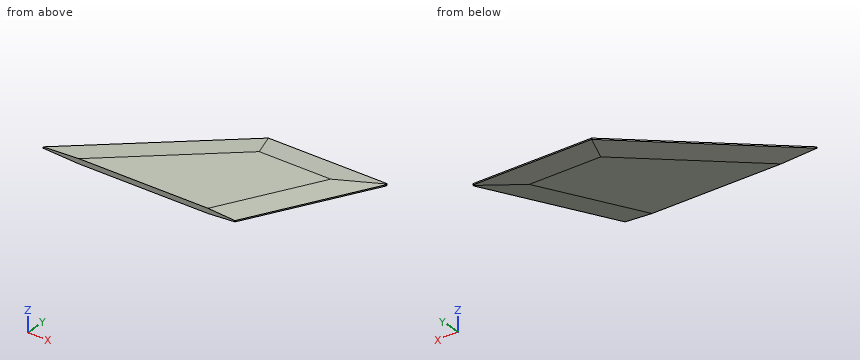
from build123d import *
from OCP.BRepFilletAPI import BRepFilletAPI_MakeChamfer

# Parameters (mm, degrees)
BOSS_EXTRUDE1_DEPTH = 1
CHAMFER1_SIZE       = 0.75
CHAMFER1_SIZE2      = 10
FILLET1_R           = 0.5


# Read off the part's stored shape, not the designer's step: Mirror1
with BuildPart() as part:
    # Sketch1 → Boss-Extrude1 (new, symmetric)
    with BuildSketch(Plane.XY):
        Polygon((0, 0), (80, 0), (105.530625741, 50), (55.530625741, 50), align=None)
    extrude(amount=BOSS_EXTRUDE1_DEPTH, both=True)

    # Chamfer1: one chamfer whose edges measure the first distance from different faces: ONE call of the kernel's chamfer builder (chamfer() names one face for all edges)
    chamfer1_edges_1 = [part.edges().sort_by_distance(p)[0] for p in [
        (92.765312871, 25, 1),
    ]]
    chamfer1_side_1 = [part.faces().sort_by_distance(p)[0] for p in [
        (92.765312871, 25, 0),
    ]]
    chamfer1_edges_2 = [part.edges().sort_by_distance(p)[0] for p in [
        (80.530625741, 50, 1),
    ]]
    chamfer1_side_2 = [part.faces().sort_by_distance(p)[0] for p in [
        (80.530625741, 50, 0),
    ]]
    chamfer1_edges_3 = [part.edges().sort_by_distance(p)[0] for p in [
        (27.765312871, 25, 1),
    ]]
    chamfer1_side_3 = [part.faces().sort_by_distance(p)[0] for p in [
        (27.765312871, 25, 0),
    ]]
    chamfer1 = BRepFilletAPI_MakeChamfer(part.part.solid().wrapped)
    for e in chamfer1_edges_1:
        chamfer1.Add(CHAMFER1_SIZE, CHAMFER1_SIZE2, e.wrapped, chamfer1_side_1[0].wrapped)  # the first distance lies on this face
    for e in chamfer1_edges_2:
        chamfer1.Add(CHAMFER1_SIZE, CHAMFER1_SIZE2, e.wrapped, chamfer1_side_2[0].wrapped)  # the first distance lies on this face
    for e in chamfer1_edges_3:
        chamfer1.Add(CHAMFER1_SIZE, CHAMFER1_SIZE2, e.wrapped, chamfer1_side_3[0].wrapped)  # the first distance lies on this face
    add(Compound.cast(chamfer1.Shape()), mode=Mode.REPLACE)

    # Mirror1
    split(bisect_by=Plane.XY, keep=Keep.TOP)

    # Mirror1 2: part across plane


with BuildPart() as part_1:
    add(part.part)
    add(part.part.mirror(Plane.XY))

    # Fillet1
    fillet1_edges = [part_1.edges().sort_by_distance(p)[0] for p in [
        (55.530625741, 50, 0),
        (105.530625741, 50, 0),
    ]]
    fillet(fillet1_edges, radius=FILLET1_R)


solid = part_1.part
The listing builds one solid part. Answer for the finished solid, in the listing's coordinates (mm). Coordinates: 2 decimals unless noted, no trailing zeros. Order: outer loops, then holes, each group sorted by start corner. A loop starts at its lowest first (then second) coordinate and runs counter-clockwise, first axis right, second up. Notation, with made-up numbers: (83, 2.5) -> (124, 2.5) arc R22 ccw to (124, 40.5) -> close; hole circle Ø11 at (65.5, 16.25). An arc over 180 degrees is marked (long way). Answer in a Markdown table with one row per item. Add a question column.
Item 1: Find section A-A (x = 72.5). Write down the section's boundary in (y, z).
Item 2: This flat-tipped pin is pushed along its axis until it touches: P1, Ø12, axis at x = 12.5, y = 14.5, coming from the -Z side. Where does it stop, or does it pass through?
Item 3: Find section D-D (x = 93.5). Write down the section's boundary in (y, z), then the cut area to 3 significant figures.
Item 4: Find section B-B (y = 31.5). Write down the section's boundary in (x, z), then the cut area to 3 significant figures.
Item 5: Find section C-C (z = -0.6). Write down the section's boundary in (x, y).
Item 6: Find the intervals of material crossed by L1, parallel to Y at x = 95, z = 0.2; L2, parallel to Y at x = 22, z = 0.1; L3, parallel to Z at x = 48, y = 39.5, in increasing order. Write a range as from..to.
Result set:
| question | item | result |
|---|---|---|
| 1 | outline | (0, -0.75) -> (7.3, -1) -> (40, -1) -> (50, -0.25) -> (50, 0.25) -> (40, 1) -> (7.3, 1) -> (0, 0.75) -> close |
| 2 | P1 | stops at z = -0.52 |
| 3 | outline | (26.44, -0.25) -> (42.63, -0.8) -> (50, -0.25) -> (50, 0.25) -> (42.63, 0.8) -> (26.44, 0.25) -> close |
| 3 | area | 24.8 mm² |
| 4 | outline | (34.98, -0.25) -> (49.93, -1) -> (84.86, -1) -> (96.08, -0.25) -> (96.08, 0.25) -> (84.86, 1) -> (49.93, 1) -> (34.98, 0.25) -> close |
| 4 | area | 103 mm² |
| 5 | outline | (6.97, 0) -> (74.76, 0) -> (97.91, 45.33) -> (57.32, 45.33) -> close |
| 6 | L1 | y = 29.38..50 |
| 6 | L2 | y = 0..19.81 |
| 6 | L3 | z = -0.46..0.46 |
